from build123d import *

# Parameters (mm, degrees)
SKETCH1_R               = 4
BOSS_EXTRUDE1_DEPTH     = 7
BOSS_EXTRUDE1_2_DEPTH   = 7
BOSS_EXTRUDE1_3_DEPTH   = 7
BOSS_EXTRUDE1_4_DEPTH   = 7
BOSS_EXTRUDE1_5_DEPTH   = 7
BOSS_EXTRUDE1_6_DEPTH   = 7
BOSS_EXTRUDE2_OUTLINE_R = 1.700000005
BOSS_EXTRUDE2_DEPTH     = 18
SKETCH2_W               = 2.2
SKETCH2_H               = 5.00000001
BOSS_EXTRUDE3_DEPTH     = 6
CUT_EXTRUDE1_DEPTH      = 1


# Read off the part's stored shape, not the designer's step: Boss-Extrude2
with BuildPart() as part:
    # Sketch1 → Boss-Extrude1 (new body)
    with BuildSketch(Plane(origin=(0, 0, 0), x_dir=(1, 0, 0), z_dir=(0, 1, 0))):
        Polygon((3.686387934, -16.664883738), (3.686388262, -4.664883738), (-8.313611738, -4.66488341), (-8.313612066, -16.66488341), align=None)
        with Locations(Location((-2.313611902, -10.664883574, 0), (0, 0, 270))):
            Circle(SKETCH1_R, mode=Mode.SUBTRACT)
    extrude(amount=BOSS_EXTRUDE1_DEPTH)



with BuildPart() as body_2:
    # Sketch1 → Boss-Extrude1 2 (new body)
    with BuildSketch(Plane(origin=(0, 0, 0), x_dir=(1, 0, 0), z_dir=(0, 1, 0))):
        Polygon((19.086387939, -16.664884095), (19.086388267, -4.664884095), (7.086388267, -4.664883767), (7.086387939, -16.664883767), align=None)
        with Locations(Location((13.086388103, -10.664883931, 0), (0, 0, 270))):
            Circle(SKETCH1_R, mode=Mode.SUBTRACT)
    extrude(amount=BOSS_EXTRUDE1_2_DEPTH)


with BuildPart() as body_3:
    # Sketch1 → Boss-Extrude1 3 (new body)
    with BuildSketch(Plane(origin=(0, 0, 0), x_dir=(1, 0, 0), z_dir=(0, 1, 0))):
        Polygon((34.486387949, -16.66488445), (34.486388277, -4.66488445), (22.486388277, -4.664884122), (22.486387949, -16.664884122), align=None)
        with Locations(Location((28.486388113, -10.664884286, 0), (0, 0, 270))):
            Circle(SKETCH1_R, mode=Mode.SUBTRACT)
    extrude(amount=BOSS_EXTRUDE1_3_DEPTH)


with BuildPart() as body_4:
    # Sketch1 → Boss-Extrude1 4 (new body)
    with BuildSketch(Plane(origin=(0, 0, 0), x_dir=(1, 0, 0), z_dir=(0, 1, 0))):
        Polygon((14.786387887, -17.664883977), (14.786387559, -29.664883977), (26.786387559, -29.664884305), (26.786387887, -17.664884305), align=None)
        with Locations(Location((20.786387723, -23.664884141, 0), (0, 0, 270))):
            Circle(SKETCH1_R, mode=Mode.SUBTRACT)
    extrude(amount=BOSS_EXTRUDE1_4_DEPTH)


with BuildPart() as body_5:
    # Sketch1 → Boss-Extrude1 5 (new body)
    with BuildSketch(Plane(origin=(0, 0, 0), x_dir=(1, 0, 0), z_dir=(0, 1, 0))):
        Polygon((30.186386338, -17.664884333), (30.18638601, -29.664884333), (42.18638601, -29.664884661), (42.186386338, -17.664884661), align=None)
        with Locations(Location((36.186386174, -23.664884497, 0), (0, 0, 270))):
            Circle(SKETCH1_R, mode=Mode.SUBTRACT)
    extrude(amount=BOSS_EXTRUDE1_5_DEPTH)


with BuildPart() as body_6:
    # Sketch1 → Boss-Extrude1 6 (new body)
    with BuildSketch(Plane(origin=(0, 0, 0), x_dir=(1, 0, 0), z_dir=(0, 1, 0))):
        Polygon((-0.613612103, -17.664883618), (-0.613612431, -29.664883618), (11.386387569, -29.664883947), (11.386387897, -17.664883947), align=None)
        with Locations(Location((5.386387733, -23.664883782, 0), (0, 0, 270))):
            Circle(SKETCH1_R, mode=Mode.SUBTRACT)
    extrude(amount=BOSS_EXTRUDE1_6_DEPTH)


with BuildPart() as part_1:
    add(part.part)

    add(body_2.part)  # Boss-Extrude2 merges body 2

    add(body_3.part)  # Boss-Extrude2 merges body 3

    add(body_4.part)  # Boss-Extrude2 merges body 4

    add(body_5.part)  # Boss-Extrude2 merges body 5

    add(body_6.part)  # Boss-Extrude2 merges body 6
    # Boss-Extrude2 outline → Boss-Extrude2 (add)
    with BuildSketch(Plane(origin=(0, 0, 0), x_dir=(1, 0, 0), z_dir=(0, 1, 0))):
        Polygon((10.586388267, -4.664883862), (10.586388281, -4.164883862), (0.186388276, -4.164883578), (0.186388262, -4.664883642), (3.686388262, -4.664883738), (3.686387934, -16.664883738), (-8.313612066, -16.66488341), (-8.313611738, -4.66488341), (-4.813611731, -4.664883505), (-4.813611724, -4.164883505), (-19.06361173, -4.164883116), (-19.06361244, -30.164883114), (2.886387555, -30.164883714), (2.886387569, -29.664883714), (-0.613612431, -29.664883618), (-0.613612103, -17.664883618), (11.386387897, -17.664883947), (11.386387569, -29.664883947), (7.886387562, -29.664883851), (7.886387555, -30.164883851), (18.286387545, -30.164884073), (18.286387559, -29.664884073), (14.786387559, -29.664883977), (14.786387887, -17.664883977), (26.786387887, -17.664884305), (26.786387559, -29.664884305), (23.286387552, -29.66488421), (23.286387545, -30.16488421), (33.686385997, -30.164884494), (33.68638601, -29.664884428), (30.18638601, -29.664884333), (30.186386338, -17.664884333), (42.186386338, -17.664884661), (42.18638601, -29.664884661), (38.686386004, -29.664884565), (38.686385997, -30.164884565), (52.93638756, -30.164884954), (52.93638827, -4.164885084), (30.986388291, -4.164884354), (30.986388277, -4.664884354), (34.486388277, -4.66488445), (34.486387949, -16.66488445), (22.486387949, -16.664884122), (22.486388277, -4.664884122), (25.986388284, -4.664884218), (25.986388291, -4.164884218), (15.586388281, -4.164884108), (15.586388267, -4.664883999), (19.086388267, -4.664884095), (19.086387939, -16.664884095), (7.086387939, -16.664883767), (7.086388267, -4.664883767), align=None)
        with Locations((47.936387915, -17.164884883)):
            Circle(BOSS_EXTRUDE2_OUTLINE_R, mode=Mode.SUBTRACT)
        with Locations((-14.063612085, -17.164883252)):
            Circle(BOSS_EXTRUDE2_OUTLINE_R, mode=Mode.SUBTRACT)
    extrude(amount=BOSS_EXTRUDE2_DEPTH)

    # Sketch2 → Boss-Extrude3 (add)
    with BuildSketch(Plane.XZ):
        Polygon((10.586387955, 19.664883873), (10.586388061, 14.664883862), (8.386388061, 14.664883816), (8.386387955, 19.664883826), align=None)
        Polygon((25.986387967, 19.664884228), (25.986388072, 14.664884218), (23.786388072, 14.664884171), (23.786387967, 19.664884182), align=None)
        Polygon((33.186387781, 19.664884438), (33.186387947, 14.664884428), (30.986387947, 14.664884354), (30.986387781, 19.664884365), align=None)
        Polygon((17.786387957, 19.664884055), (17.786388062, 14.664884045), (15.586388062, 14.664883999), (15.586387957, 19.664884009), align=None)
        with Locations((1.286388276, 17.164883628)):
            Rectangle(SKETCH2_W, SKETCH2_H)
    extrude(amount=BOSS_EXTRUDE3_DEPTH)

    # Sketch3 → Cut-Extrude1 (cut)
    # profile 1 of 2: a face of its own
    with BuildSketch(Plane.XZ):
        Polygon((-8.682133254, 26.826855078), (-7.135338382, 26.826855078), (-7.135338382, 26.501214052), (-8.397197357, 26.501214052), (-8.397197357, 25.524290975), (-7.135338382, 25.524290975), (-7.135338382, 25.198649949), (-8.397197357, 25.198649949), (-8.397197357, 23.651855078), (-8.682133254, 23.651855078), align=None)
    # profile 2 of 2: a face of its own
    with BuildSketch(Plane.XZ):
        Polygon((-5.117254448, 26.908265334), (-5.059376844, 26.908265334), (-5.059376844, 24.710188411), (-4.69303069, 24.710188411), (-4.69303069, 24.384547385), (-5.059376844, 24.384547385), (-5.059376844, 23.651855078), (-5.344312741, 23.651855078), (-5.344312741, 24.384547385), (-6.850402485, 24.384547385), align=None)
        Polygon((-5.344312741, 24.710188411), (-5.344312741, 26.087802594), (-6.290070954, 24.710188411), align=None, mode=Mode.SUBTRACT)
    extrude(amount=-CUT_EXTRUDE1_DEPTH, mode=Mode.SUBTRACT)


solid = part_1.part
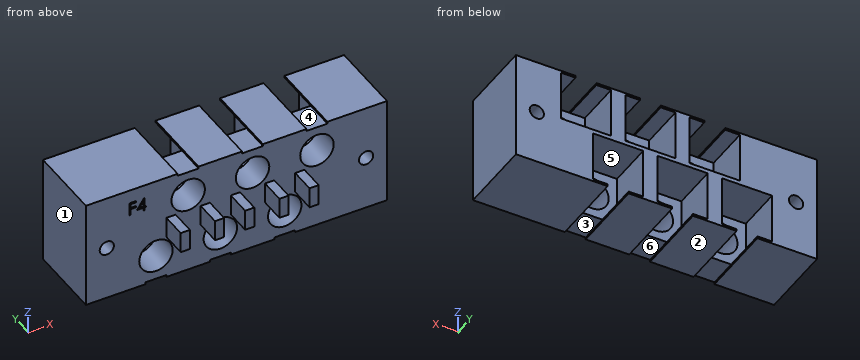
Input: part model. Units: mm. Frame: model coordinates. Face numbers are marked on the shaded views. A direction names the side the tool comes from. Round coordinates to 2 decimals unless told otherwise and drop trailing zeros. Order: outer loops, then holes, each group sorted by start corner. A loop starts at its lowest first (then second) coordinate and runs counter-clockwise, first axis right, second up. Notation, with made-up numbers: (2, 24.5) - (26, 24.5) arc R27 ccw to (26, 48.5) - close; hole circle Ø4 at (88, -25). An arc over 180 degrees is marked (long way). Answer as a JSON object with one key per item and string values. Group by question number.
(1) Material intervals for probe 1 along X at (y, z) = (10.5, 19); probe 2 along Z at (x, y) = (25.5, 17.25); probe 3 along X at (y, z) = (2.25, 23.5), sorted ascending. Write a range as from..to.
(2) Cut plane B-B (z = 9.75). Return loops of the section in (x, y), then the cut area to 3 significant figures.
(3) Cut plane D-D (z = 6). Return loops of the section in (x, y).
(4) Cut plane A-A (y = -2.5). Return loops of the section in (x, z).
(5) Reachability of the marked faces 4, 5 and 6 from +Z, -Z, +X, -X, +Y, -Y: full face, straight path, thin tool, end or side. Return the list, or none.
(6) Pin query (flat end, axial travel): P1, Ø3.5, axis at x = 38.5, z = 22, coming from the +Y side; P2, Ø2.5, axis at x = 9, y = -2.5, coming from the +Z side; P3, Ø2.5, axis at y = -2, z = 16.5, coming from the +X side; P4, Ø4, axis at x = -6, y = -3.5, coming from the +Z side. Return the tip coordinate at first contact, or that it passes through.
(7) Draft query along X for the marked faces 1, 2 and 3. Return one class per face: released by +X, released by -X, zero draft, split by the parting line, or undercut.
(8) Cut plane C-C (x = -3.5). Return loops of the section in (y, z), then the cut area to 3 significant figures.
Here are the results:
{
 "1": {"probe 1": "x = -19.06..-0.61, 11.39..14.79, 26.79..30.19, 42.19..52.94", "probe 2": "z = 4.16..4.66, 16.66..17.66, 29.66..30.16", "probe 3": "x = -19.06..1.39, 9.38..16.79, 24.78..32.19, 40.18..52.94"},
 "2": {"outline": "(-19.06, 0) - (-6.21, 0) - (-6.21, 7) - (-8.31, 7) - (-8.31, 18) - (-19.06, 18) - close; (1.58, 0) - (9.19, 0) - (9.19, 7) - (7.09, 7) - (7.09, 18) - (3.69, 18) - (3.69, 7) - (1.58, 7) - close; (16.98, 0) - (24.59, 0) - (24.59, 7) - (22.49, 7) - (22.49, 18) - (19.09, 18) - (19.09, 7) - (16.98, 7) - close; (32.38, 0) - (52.94, 0) - (52.94, 18) - (34.49, 18) - (34.49, 7) - (32.38, 7) - close", "area": "736 mm^2"},
 "3": {"outline": "(-19.06, 0) - (52.94, 0) - (52.94, 18) - (34.49, 18) - (34.49, 7) - (22.49, 7) - (22.49, 18) - (19.09, 18) - (19.09, 7) - (7.09, 7) - (7.09, 18) - (3.69, 18) - (3.69, 7) - (-8.31, 7) - (-8.31, 18) - (-19.06, 18) - close"},
 "4": {"outline": "(0.19, 14.66) - (2.39, 14.66) - (2.39, 19.66) - (0.19, 19.66) - close; (8.39, 14.66) - (10.59, 14.66) - (10.59, 19.66) - (8.39, 19.66) - close; (15.59, 14.66) - (17.79, 14.66) - (17.79, 19.66) - (15.59, 19.66) - close; (23.79, 14.66) - (25.99, 14.66) - (25.99, 19.66) - (23.79, 19.66) - close; (30.99, 14.66) - (33.19, 14.66) - (33.19, 19.66) - (30.99, 19.66) - close"},
 "5": {"face 4": "+Z, +Y, -Y", "face 5": "+Y", "face 6": "-Z, +Y, -Y"},
 "6": {"P1": "stops at y = 7", "P2": "stops at z = 19.66", "P3": "stops at x = 33.19", "P4": "passes through"},
 "7": {"face 1": "released by -X", "face 2": "zero draft", "face 3": "undercut"},
 "8": {"outline": "(0, 4.66) - (7, 4.66) - (7, 6.84) - (0, 6.84) - close; (0, 14.48) - (7, 14.48) - (7, 16.66) - (18, 16.66) - (18, 30.16) - (0, 30.16) - close", "area": "274 mm^2"}
}
